Geometry check sheet. Reference: the model listing, model coordinates, mm. Face numbers are marked on the shaded views. A direction names the side the tool comes from. Round coordinates to 2 decimals unless told otherwise and drop trailing zeros. Order: outer loops, then holes, each group sorted by start corner. A loop starts at its lowest first (then second) coordinate and runs counter-clockwise, first axis right, second up.
(1) Sectioned sample at A-A (z = 3.25). Record the boundary of the cut face in (x, y) (3 decimals), plus the area to 3 significant figures.
(2) Set-up check for the marked faces 5 and 6: record each of +Z, -Z, +X, -X, +Y, -Y from which the full face is reachable in a straight line by a thin tool's end or side.
(3) Release check for a two-part mould opening along Z. For the marked faces 1, 2, 3 and 4 record: +Z half, -Z half, draft (parallel to the pull), parting line (faces both ways), or undercut.
(4) Sectioned sample at C-C (y = -3). Record the boundary of the cut face in (x, z), plus the area to 3 significant figures.
(5) Sectioned sample at B-B (x = -13.5). Record the boundary of the cut face in (y, z) (3 decimals), plus the area to 3 significant figures.
(6) Sectioned sample at D-D (x = -7.75). Record the boundary of the cut face in (y, z) (3 decimals), plus the area to 3 significant figures.
(7) Go/stop test with flat-tipped pins: pin 1 (3.5 mm diameter, centred on x = -18.36, z = 3.25, fed in from +Y) (3 decimals); pin 2 (2 mm diameter, centred on y = -1.5, z = 2, fed in from -X). Record where each tip stops, or that it passes through.
(8) Material ranges on line 1 along X through (y, z) = (-4.3, 3.25); line 2 along Y through (x, z) = (-7.2, 3.25) (3 decimals); line 3 along X through (y, z) = (-1.25, 5.75), recorded low to high.
from build123d import *

# Parameters (mm, degrees)
BOSS_EXTRUDE1_DEPTH = 6.5
SKETCH2_R           = 1.55
CUT_EXTRUDE1_DEPTH  = 10
SKETCH3_R           = 1.55
CUT_EXTRUDE2_DEPTH  = 10


with BuildPart() as part:
    # Sketch1 → Boss-Extrude1 (new body)
    with BuildSketch(Plane.XY):
        Polygon((-21.361853088, -2.625), (-9.361853088, -2.625), (-9.361853088, 17.375), (-6.361853088, 17.375), (-6.361853088, -5.625), (-9.361853088, -5.625), (-21.361853088, -5.625), align=None)
    extrude(amount=BOSS_EXTRUDE1_DEPTH)

    # Sketch2 → Cut-Extrude1 (cut)
    with BuildSketch(Plane(origin=(0, -2.625, 0), x_dir=(1, 0, 0), z_dir=(0, 1, 0))):
        with Locations(Location((-12.361853088, -3.25, 0), (0, 0, 270))):
            Circle(SKETCH2_R)
        with Locations(Location((-18.361853088, -3.25, 0), (0, 0, 270))):
            Circle(SKETCH2_R)
    extrude(amount=-CUT_EXTRUDE1_DEPTH, mode=Mode.SUBTRACT)

    # Sketch3 → Cut-Extrude2 (cut)
    with BuildSketch(Plane.ZY.offset(9.361853088)):
        with Locations((3.25, 1.725)):
            Circle(SKETCH3_R)
        with Locations((3.25, 11.025)):
            Circle(SKETCH3_R)
    extrude(amount=-CUT_EXTRUDE2_DEPTH, mode=Mode.SUBTRACT)


solid = part.part
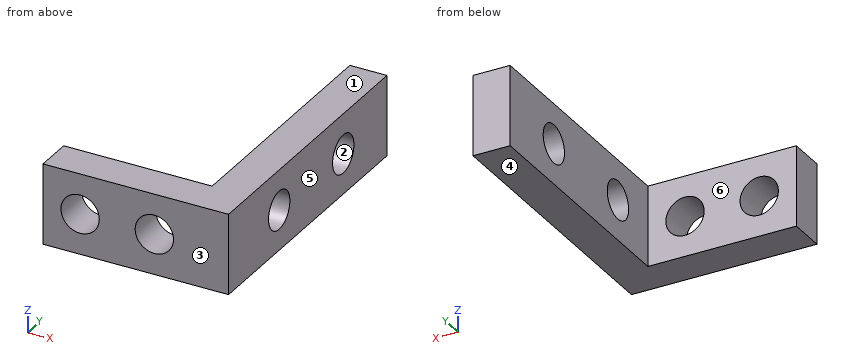
Answer below:
1. outline: (-21.362, -5.625) - (-19.912, -5.625) - (-19.912, -2.625) - (-21.362, -2.625) - close; (-16.812, -5.625) - (-13.912, -5.625) - (-13.912, -2.625) - (-16.812, -2.625) - close; (-10.812, -5.625) - (-6.362, -5.625) - (-6.362, 0.175) - (-9.362, 0.175) - (-9.362, -2.625) - (-10.812, -2.625) - close; (-9.362, 3.275) - (-6.362, 3.275) - (-6.362, 9.475) - (-9.362, 9.475) - close; (-9.362, 12.575) - (-6.362, 12.575) - (-6.362, 17.375) - (-9.362, 17.375) - close
1. area: 67.8 mm2
2. face 5: +Z, -Z, +X, +Y, -Y
2. face 6: +Z, -Z, -X, +Y
3. face 1: +Z half
3. face 2: undercut
3. face 3: draft
3. face 4: -Z half
4. outline: (-21.36, 0) - (-6.36, 0) - (-6.36, 6.5) - (-21.36, 6.5) - close; hole circle Ø3.1 at (-18.36, 3.25); hole circle Ø3.1 at (-12.36, 3.25)
4. area: 82.4 mm2
5. outline: (-5.625, 0) - (-2.625, 0) - (-2.625, 2.198) - (-5.625, 2.198) - close; (-5.625, 4.302) - (-2.625, 4.302) - (-2.625, 6.5) - (-5.625, 6.5) - close
5. area: 13.2 mm2
6. outline: (-5.625, 0) - (17.375, 0) - (17.375, 6.5) - (-5.625, 6.5) - close; hole circle Ø3.1 at (1.725, 3.25); hole circle Ø3.1 at (11.025, 3.25)
6. area: 134 mm2
7. pin 1: stops at y = -2.625
7. pin 2: stops at x = -9.36
8. line 1: x = -21.36 to -19.91, -16.81 to -13.91, -10.81 to -6.36
8. line 2: y = -5.625 to 0.175, 3.275 to 9.475, 12.575 to 17.375
8. line 3: x = -9.36 to -6.36
